The listing builds one solid part. Answer for the finished solid, in the listing's coordinates (mm). A direction names the side the tool comes from. Give positions to 0.01 mm unless a question says otherwise; leave off trailing zeros. Loops run counter-clockwise (first coordinate to the right, second up) from the corner with the lowest first, then second, coordinate; pieces in that order, holes last. Notation, with made-up numbers: M 50,-14 L 74,-14 A20 cw 74,23 Z; hole C -31.5,62 d6. An arc over 180 degrees is marked long. One line per item, written item: value. Start each with the question number.
Q1. A cutting plane is placed at B-B, the plane y = 5. Determine the outline of the cut face in (x, z).
Q2. A cutting plane is placed at A-A, the plane z = -28. Determine the outline of the cut face in (x, y).
Q3. The mould has two halves that part along X. Classify faces 1 (the flat face through (15, 3, -18)), 2 (the flat face through (-3, 4, -33)), 3 (the flat face through (32, 4, -21)), 4 (the flat face through (0, 5, -33)): +X half, -X half, draft (parallel to the pull), parting line (faces both ways), or undercut.
Q4. Flat-ended cylindrical pins translate along their axes: pin 1 (3 mm diameter, centred on y = 5, z = -7.5, fed in from -X); pin 2 (0.9 mm diameter, centred on x = 31.5, y = 3.5, fed in from +Z); pin 3 (2.5 mm diameter, centred on y = 1, z = -14, fed in from +X); pin 4 (9 mm diameter, centred on x = 12, z = -25, fed in from +Y). Find the tip coordinate at first contact, or state that the pin passes through.
Q5. A cutting plane is placed at C-C, the plane x = 25.5. Determine the outline of the cut face in (y, z).
Q6. A cutting plane is placed at D-D, the plane y = 1.75. Determine the outline of the cut face in (x, z).
Q7. For faces 5 (the cylindrical face through (25.46, 7.93, -42.15)), 6 (the flat face through (30, 1, -11)), 7 (the flat face through (23.5, 1, -33)), 8 (the flat face through (0, 1, -10)), determine the directions among +Z, -Z, +X, -X, +Y, -Y from which every point of the face is accessible in a straight line to the end or side of a thin tool.
Q8. Consider L1, parallel to X at y = 6.5, z = -38; L2, parallel to Y at x = 8, z = -6; L3, parallel to Z at x = 8.5, y = 2.25. Determine where each line is inside the solid, lowest interval first.
from build123d import *

# Parameters (mm, degrees)
BOSS_EXTRUDE1_DEPTH = 3
SKETCH2_R           = 0.85
SKETCH2_W           = 3
SKETCH2_H           = 24
BOSS_EXTRUDE2_DEPTH = 5
SKETCH3_R           = 0.85
BOSS_EXTRUDE3_DEPTH = 5


with BuildPart() as part:
    # Sketch1 → Boss-Extrude1 (new body)
    with BuildSketch(Plane(origin=(0, 0, 0), x_dir=(1, 0, 0), z_dir=(0, 1, 0))):
        Polygon((30, 0), (0, 0), (0, 21), (-3, 21), (-3, 45), (6.5, 45), (6.5, 21), (23.5, 21), (23.5, 45), (33, 45), (33, 21), (30, 21), align=None)
    extrude(amount=BOSS_EXTRUDE1_DEPTH)

    # Sketch2 → Boss-Extrude2 (add)
    with BuildSketch(Plane(origin=(0, 3, 0), x_dir=(1, 0, 0), z_dir=(0, 1, 0))):
        with Locations(Location((4.5, 43, 0), (0, 0, 90))):
            Circle(SKETCH2_R)
        with Locations(Location((25.5, 43, 0), (0, 0, 90))):
            Circle(SKETCH2_R)
        with Locations(Location((25.5, 30.5, 0), (0, 0, 90))):
            Circle(SKETCH2_R)
        with Locations(Location((4.5, 30.5, 0), (0, 0, 90))):
            Circle(SKETCH2_R)
        with Locations((-1.5, 33)):
            Rectangle(SKETCH2_W, SKETCH2_H)
        with Locations((31.5, 33)):
            Rectangle(SKETCH2_W, SKETCH2_H)
    extrude(amount=BOSS_EXTRUDE2_DEPTH)

    # Sketch3 → Boss-Extrude3 (add)
    with BuildSketch(Plane(origin=(0, 8, 0), x_dir=(1, 0, 0), z_dir=(0, 1, 0))):
        with Locations(Location((4.5, 43, 0), (0, 0, 90))):
            Circle(SKETCH3_R)
        with Locations(Location((25.5, 43, 0), (0, 0, 90))):
            Circle(SKETCH3_R)
        with Locations(Location((25.5, 30.5, 0), (0, 0, 90))):
            Circle(SKETCH3_R)
        with Locations(Location((4.5, 30.5, 0), (0, 0, 90))):
            Circle(SKETCH3_R)
    extrude(amount=BOSS_EXTRUDE3_DEPTH)


solid = part.part
Answer block:
1. outline: M -3,-45 L 0,-45 L 0,-21 L -3,-21 Z; C 4.5,-43 d1.7; C 4.5,-30.5 d1.7; C 25.5,-43 d1.7; C 25.5,-30.5 d1.7; M 30,-45 L 33,-45 L 33,-21 L 30,-21 Z
2. outline: M -3,0 L 6.5,0 L 6.5,3 L 0,3 L 0,8 L -3,8 Z; M 23.5,0 L 33,0 L 33,8 L 30,8 L 30,3 L 23.5,3 Z
3. face 1: undercut
3. face 2: -X half
3. face 3: draft
3. face 4: undercut
4. pin 1: through
4. pin 2: z = -21
4. pin 3: x = 30
4. pin 4: y = 3
5. outline: M 0,-45 L 3,-45 L 3,-43.85 L 13,-43.85 L 13,-42.15 L 3,-42.15 L 3,-31.35 L 13,-31.35 L 13,-29.65 L 3,-29.65 L 3,0 L 0,0 Z
6. outline: M -3,-45 L 6.5,-45 L 6.5,-21 L 23.5,-21 L 23.5,-45 L 33,-45 L 33,-21 L 30,-21 L 30,0 L 0,0 L 0,-21 L -3,-21 Z
7. face 5: +Y
7. face 6: +Z, +X, +Y, -Y
7. face 7: -Z, +Y, -Y
7. face 8: +Z, -X, +Y, -Y
8. L1: -3 to 0, 30 to 33
8. L2: 0 to 3
8. L3: -21 to 0
